from build123d import *

# Parameters (mm, degrees)
F0_R     = 1.5875
F0_R_2   = 4.318
F1_DEPTH = 3.175
F3_DEPTH = 2.032
F5_R     = 4.318
F6_DEPTH = 2.54


with BuildPart() as f1:
    # F0 (on Top) → F1 (new body)
    with BuildSketch(Plane.XY):
        Polygon((11.049, -6.379143), (11.049, 6.379143), (0, 12.758286), (-11.049, 6.379143), (-11.049, -6.379143), (0, -12.758286), align=None)
        with Locations((-8.248892, -4.7625)):
            Circle(F0_R, mode=Mode.SUBTRACT)
        with Locations((8.248892, -4.7625)):
            Circle(F0_R, mode=Mode.SUBTRACT)
        Circle(F0_R_2, mode=Mode.SUBTRACT)
        with Locations((0, 9.525)):
            Circle(F0_R, mode=Mode.SUBTRACT)
    extrude(amount=F1_DEPTH)

    # F2 (on face) → F3 (cut)
    with BuildSketch(Plane.XY.offset(3.175)):
        with BuildLine():
            Line((0, 12.758286), (-3.984707, 10.457715))
            Line((-3.984707, 10.457715), (-2.584653, 8.03275))
            ThreePointArc((-2.584653, 8.03275), (0, 6.5405), (2.584653, 8.03275))
            Line((2.584653, 8.03275), (3.984707, 10.457715))
            Line((3.984707, 10.457715), (0, 12.758286))
        make_face()
        with BuildLine():
            Line((-8.248892, -1.778), (-11.049, -1.778))
            Line((-11.049, -1.778), (-11.049, -6.379143))
            Line((-11.049, -6.379143), (-7.064293, -8.679715))
            Line((-7.064293, -8.679715), (-5.664239, -6.25475))
            ThreePointArc((-5.664239, -6.25475), (-5.664239, -3.27025), (-8.248892, -1.778))
        make_face()
        with BuildLine():
            Line((5.664239, -6.25475), (7.064293, -8.679715))
            Line((7.064293, -8.679715), (11.049, -6.379143))
            Line((11.049, -6.379143), (11.049, -1.778))
            Line((11.049, -1.778), (8.248892, -1.778))
            ThreePointArc((8.248892, -1.778), (5.664239, -3.27025), (5.664239, -6.25475))
        make_face()
    extrude(amount=-F3_DEPTH, mode=Mode.SUBTRACT)

    # F5 (on face) → F6 (join)
    with BuildSketch(Plane.XY.offset(3.175)):
        with BuildLine():
            ThreePointArc((-6.60542, -2.271268), (-5.664239, -3.27025), (-5.269685, -4.584827))
            ThreePointArc((-5.269685, -4.584827), (0, -6.985), (5.269685, -4.584827))
            ThreePointArc((5.269685, -4.584827), (5.664239, -3.27025), (6.60542, -2.271268))
            ThreePointArc((6.60542, -2.271268), (6.049187, 3.4925), (1.335734, 6.856095))
            ThreePointArc((1.335734, 6.856095), (0, 6.5405), (-1.335734, 6.856095))
            ThreePointArc((-1.335734, 6.856095), (-6.049187, 3.4925), (-6.60542, -2.271268))
        make_face()
        Circle(F5_R, mode=Mode.SUBTRACT)
    extrude(amount=F6_DEPTH)


solid = f1.part
Here's how the part is built. I have some questions about the finished solid (model axes, mm). A direction names the side the tool comes from. Give positions to 0.01 mm unless a question says otherwise; leave off trailing zeros. Loops run counter-clockwise (first coordinate to the right, second up) from the corner with the lowest first, then second, coordinate; pieces in that order, holes last. Notation, with made-up numbers: (34.5, 9) -> (51.5, 9) arc R17 ccw to (51.5, 34) -> close; hole circle Ø4 at (66, -28.75). An arc over 180 degrees is marked (long way). Answer as a JSON object with one key per item and string values. Group by question number.
Item 1: I need wall thicknesses on L1, parallel to X at y = -2, z = 4.7; L2, parallel to Y at x = -8.75, z = 0.35; L3, parallel to X at y = -2.25, z = 3.9. Which ranges of each line are inside material? Lowest first, please.
Item 2: Imagine slicing it at B-B on z = 3.8. Write out the boundary of the cut face in (x, y) (1 decimal), then the cut area to 3 significant figures.
Item 3: Imagine slicing it at C-C on x = 2. Write out the boundary of the cut face in (y, z) (3 decimals).
Item 4: Imagine slicing it at D-D on z = 2.5. Write out the boundary of the cut face in (x, y) (1 decimal).
Item 5: Imagine slicing it at A-A on y = 0. Write out the boundary of the cut face in (x, z) (3 decimals), then the cut area to 3 significant figures.
Item 6: Thinking about a two-plate mould opening in Y: for faces 1 (the flat face through (2, 10, 1.143)), 2 (the flat face through (-6.675, 8.905, 1.565)), 3 (the flat face through (6.354, -7.45, 2.173)), which applies, pulls with the +Y half, pulls with the -Y half, needs draft (parallel to the pull), parting line crosses it, or undercut?
Item 7: Will these pins go through, and if not, where does the flat tip stop? pin 1 (2 mm diameter, centred on x = -10, z = 2, fed in from -Y); pin 2 (4.5 mm diameter, centred on x = 8.5, y = -4.5, fed in from +Z); pin 3 (1 mm diameter, centred on x = 0.5, z = 2, fed in from +Y).
Item 8: On a 3-axis mill with a long thin cutter (end or side, diameter ignored), from which of +Z, -Z, +X, -X, +Y, -Y can I reach the whole of each face in a straight line? I mean faces 4 (the flat face through (10, -1.778, 2)), 5 (the flat face through (-10, -1.778, 2)), 6 (the cylindrical face through (6.1, 3.4, 4.4)), 7 (the flat face through (3.275, 9.228, 2.173)). Say none if no direction works.
Answer list:
{
 "1": {"L1": "x = -6.69 to -3.83, 3.83 to 6.69", "L2": "y = -7.71 to -6.27, -3.26 to 7.71", "L3": "x = -6.61 to -3.69, 3.69 to 6.61"},
 "2": {"outline": "(-6.6, -2.3) arc R3 cw to (-5.3, -4.6) arc R7 ccw to (5.3, -4.6) arc R3 cw to (6.6, -2.3) arc R7 ccw to (1.3, 6.9) arc R3 cw to (-1.3, 6.9) arc R7 ccw to start; hole circle Ø8.6 at (0, 0)", "area": "92.3 mm2"},
 "3": {"outline": "(-11.604, 0) -> (-3.827, 0) -> (-3.827, 5.715) -> (-6.693, 5.715) -> (-6.693, 3.175) -> (-11.604, 3.175) -> close; (3.827, 0) -> (11.604, 0) -> (11.604, 1.143) -> (7.31, 1.143) -> (7.31, 3.175) -> (6.693, 3.175) -> (6.693, 5.715) -> (3.827, 5.715) -> close"},
 "4": {"outline": "(-11, -1.8) -> (-8.2, -1.8) arc R3 cw to (-5.7, -6.3) -> (-7.1, -8.7) -> (0, -12.8) -> (7.1, -8.7) -> (5.7, -6.3) arc R3 cw to (8.2, -1.8) -> (11, -1.8) -> (11, 6.4) -> (4, 10.5) -> (2.6, 8) arc R3 cw to (-2.6, 8) -> (-4, 10.5) -> (-11, 6.4) -> close; hole circle Ø8.6 at (0, 0)"},
 "5": {"outline": "(-11.049, 0) -> (-4.318, 0) -> (-4.318, 5.715) -> (-6.985, 5.715) -> (-6.985, 3.175) -> (-11.049, 3.175) -> close; (4.318, 0) -> (11.049, 0) -> (11.049, 3.175) -> (6.985, 3.175) -> (6.985, 5.715) -> (4.318, 5.715) -> close", "area": "56.3 mm2"},
 "6": {"face 1": "needs draft", "face 2": "pulls with the +Y half", "face 3": "undercut"},
 "7": {"pin 1": "stops at y = -7.28", "pin 2": "stops at z = 1.14", "pin 3": "stops at y = 6.71"},
 "8": {"face 4": "+Z, +X, -Y", "face 5": "+Z, -X, -Y", "face 6": "+Z, +X", "face 7": "+Z, +Y"}
}
